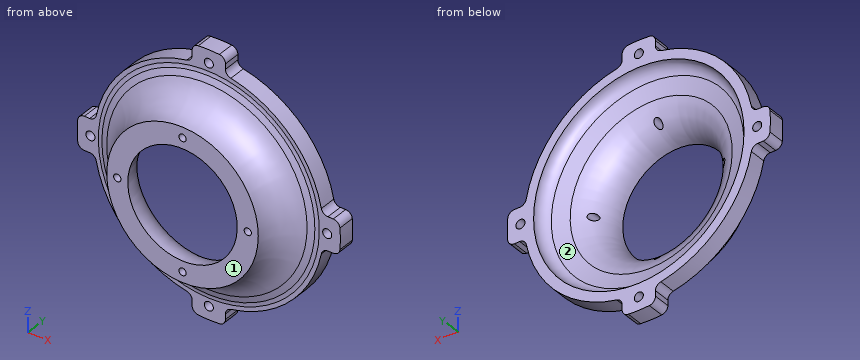
from build123d import *

# Parameters (mm, degrees)
F_18_0_1695_DIAMETER_HOLE1_D = 4.3053
F_8_32_TAPPED_HOLE1_D        = 3.4544
CUT_EXTRUDE1_START           = -28
CUT_EXTRUDE1_DEPTH           = 28


with BuildPart() as part:
    # Sketch1 → Revolve1 (revolve)
    with BuildSketch(Plane.XY, mode=Mode.PRIVATE) as revolve1_sk:
        with BuildLine():
            Line((-62.5, 25), (-62.5, 17))
            Line((-62.5, 17), (-52.5, 17))
            ThreePointArc((-52.5, 17), (-51.542432766, 16.927385203), (-50.606765862, 16.711201572))
            Line((-50.606765862, 16.711201572), (-47.596209994, 15.770845592))
            ThreePointArc((-47.596209994, 15.770845592), (-39.211088387, 9.787640892), (-36, 0))
            Line((-36, 0), (-26, 0))
            ThreePointArc((-26, 0), (-29.461355465, 10.550473923), (-38.5, 17))
            Line((-38.5, 17), (-45.792532285, 19.277843908))
            ThreePointArc((-45.792532285, 19.277843908), (-48.834916691, 21.448737727), (-50, 25))
            Line((-50, 25), (-62.5, 25))
        make_face()
    revolve(revolve1_sk.sketch.rotate(Axis((0, 0, 0), (0, 1, 0)), 270), axis=Axis((0, 0, 0), (0, 1, 0)))

    # #18 (0.1695) Diameter Hole1 (through all)
    with Locations(Plane(origin=(0, 25, 0), x_dir=(1, 0, 0), z_dir=(0, 1, 0))):
        with Locations((0, 56.25), (0, -56.25), (-56.25, 0), (56.25, 0)):
            Hole(F_18_0_1695_DIAMETER_HOLE1_D / 2)

    # #8-32 Tapped Hole1 (through all)
    with Locations(Plane(origin=(0, 0, 0), x_dir=(-1, 0, 0), z_dir=(0, -1, 0))):
        with Locations((0, 31), (0, -31), (-31, 0), (31, 0)):
            Hole(F_8_32_TAPPED_HOLE1_D / 2)

    # Sketch7 → Cut-Extrude1 (cut)
    with BuildSketch(Plane(origin=(0, 44.982495649, 0), x_dir=(1, 0, 0), z_dir=(0, 1, 0)).offset(CUT_EXTRUDE1_START)):
        with BuildLine():
            Line((-56.597564918, 7.921), (-59.13485528, 7.921))
            ThreePointArc((-59.13485528, 7.921), (-61.28824505, 7.07913898), (-62.299678972, 5))
            ThreePointArc((-62.299678972, 5), (-44.194173824, 44.194173824), (-5, 62.299678972))
            ThreePointArc((-5, 62.299678972), (-7.07913898, 61.28824505), (-7.921, 59.13485528))
            Line((-7.921, 59.13485528), (-7.921, 56.597564918))
            ThreePointArc((-7.921, 56.597564918), (-8.644467964, 54.579988714), (-10.485166883, 53.48187801))
            ThreePointArc((-10.485166883, 53.48187801), (-38.537319575, 38.537319575), (-53.48187801, 10.485166883))
            ThreePointArc((-53.48187801, 10.485166883), (-54.579988714, 8.644467964), (-56.597564918, 7.921))
        make_face()
        with BuildLine():
            Line((7.921, 56.597564918), (7.921, 59.13485528))
            ThreePointArc((7.921, 59.13485528), (7.07913898, 61.28824505), (5, 62.299678972))
            ThreePointArc((5, 62.299678972), (44.194173824, 44.194173824), (62.299678972, 5))
            ThreePointArc((62.299678972, 5), (61.28824505, 7.07913898), (59.13485528, 7.921))
            Line((59.13485528, 7.921), (56.597564918, 7.921))
            ThreePointArc((56.597564918, 7.921), (54.579988714, 8.644467964), (53.48187801, 10.485166883))
            ThreePointArc((53.48187801, 10.485166883), (38.537319575, 38.537319575), (10.485166883, 53.48187801))
            ThreePointArc((10.485166883, 53.48187801), (8.644467964, 54.579988714), (7.921, 56.597564918))
        make_face()
        with BuildLine():
            Line((56.597564918, -7.921), (59.13485528, -7.921))
            ThreePointArc((59.13485528, -7.921), (61.28824505, -7.07913898), (62.299678972, -5))
            ThreePointArc((62.299678972, -5), (44.194173824, -44.194173824), (5, -62.299678972))
            ThreePointArc((5, -62.299678972), (7.07913898, -61.28824505), (7.921, -59.13485528))
            Line((7.921, -59.13485528), (7.921, -56.597564918))
            ThreePointArc((7.921, -56.597564918), (8.644467964, -54.579988714), (10.485166883, -53.48187801))
            ThreePointArc((10.485166883, -53.48187801), (38.537319575, -38.537319575), (53.48187801, -10.485166883))
            ThreePointArc((53.48187801, -10.485166883), (54.579988714, -8.644467964), (56.597564918, -7.921))
        make_face()
        with BuildLine():
            Line((-7.921, -56.597564918), (-7.921, -59.13485528))
            ThreePointArc((-7.921, -59.13485528), (-7.07913898, -61.28824505), (-5, -62.299678972))
            ThreePointArc((-5, -62.299678972), (-44.194173824, -44.194173824), (-62.299678972, -5))
            ThreePointArc((-62.299678972, -5), (-61.28824505, -7.07913898), (-59.13485528, -7.921))
            Line((-59.13485528, -7.921), (-56.597564918, -7.921))
            ThreePointArc((-56.597564918, -7.921), (-54.579988714, -8.644467964), (-53.48187801, -10.485166883))
            ThreePointArc((-53.48187801, -10.485166883), (-38.537319575, -38.537319575), (-10.485166883, -53.48187801))
            ThreePointArc((-10.485166883, -53.48187801), (-8.644467964, -54.579988714), (-7.921, -56.597564918))
        make_face()
    extrude(amount=CUT_EXTRUDE1_DEPTH, mode=Mode.SUBTRACT)


solid = part.part
Work out the finished part from the listing and answer in its coordinate system (mm). Face numbers are marked on the shaded views. Give positions to 0.01 mm unless a question says otherwise; leave off trailing zeros. Loops run counter-clockwise (first coordinate to the right, second up) from the corner with the lowest first, then second, coordinate; pieces in that order, holes last. Notation, with made-up numbers: (-26.75, -35.75) - (-8.75, -35.75) arc R11 ccw to (-8.75, -27.75) - close; hole circle Ø6 at (43, 53). An arc over 180 degrees is marked (long way). Answer in a Markdown table with one row per item.
(1) For a pull along Z with two mould halves and no side action, classify the marked faces 1 and 2 as pulls with the +Z half, pulls with the -Z half, needs draft (parallel to the pull), parting line crosses it, or undercut.
Results list:
| item | result |
|---|---|
| face 1 | needs draft |
| face 2 | undercut |
(2) Section A-A (y = 5.25) is taken. Give the vertices of the cut face in (x, z), and give its area (3 significant figures).
Results list:
| item | result |
|---|---|
| outline | circle Ø73.71 at (0, 0); hole circle Ø3.45 at (-31, 0); hole circle Ø53.58 at (0, 0); hole circle Ø3.45 at (0, -31); hole circle Ø3.45 at (0, 31); hole circle Ø3.45 at (31, 0) |
| area | 1,980 mm² |
(3) Flat-ended cylindrical pins translate along their axes: pin 1 Ø1.3 at (x, y) = (-58.5, 20.5) entering from +Z; pin 2 Ø0.8 at (y, z) = (19.5, -58.5) entering from +X; pin 3 Ø5 at (x, z) = (0, 56.25) entering from +Y; pin 4 Ø6 at (x, y) = (18, 22) entering from -Z. Find the tip coordinate at first contact, or state that the pin passes through.
Results list:
| item | result |
|---|---|
| pin 1 | stops at z = 7.92 |
| pin 2 | stops at x = 7.92 |
| pin 3 | stops at y = 25 |
| pin 4 | stops at z = -52.4 |
(4) Section B-B (y = 23.25) is taken. State how many separate pieces and enclosed holes the cut face has, and give its area (3 significant figures).
Results list:
| item | result |
|---|---|
| separate pieces | 1 |
| enclosed holes | 5 |
| area | 2,010 mm² |
(5) Consider L1, parallel to Z at x = 1.5, y = 24; L2, parallel to Z at x = 15, y = 4.25; L3, parallel to Z at x = -43.5, y = 23. Determine where each line is inside the solid, lowest interval first. Write a range as [from, to].
Results list:
| item | result |
|---|---|
| L1 | z = [-62.48, -57.79], [-54.71, -49.89], [49.89, 54.71], [57.79, 62.48] |
| L2 | z = [-33.34, -21.86], [21.86, 33.34] |
| L3 | z = [-32.83, -23.95], [23.95, 32.83] |
